The listing builds one solid part. Answer for the finished solid, in the listing's coordinates (mm). A direction names the side the tool comes from. Coordinates: 2 decimals unless noted, no trailing zeros. Order: outer loops, then holes, each group sorted by start corner. A loop starts at its lowest first (then second) coordinate and runs counter-clockwise, first axis right, second up. Notation, with made-up numbers: (9.5, 71) -> (45.5, 71) arc R12 ccw to (45.5, 93) -> close; hole circle Ø10 at (-28.75, 57). An arc over 180 degrees is marked (long way). Answer in a Markdown table with one row per item.
```python
from build123d import *

# Parameters (mm, degrees)
BOSS_EXTRUDE1_DEPTH = 19.5
SHELL1_T            = -3
SKETCH2_W           = 36
SKETCH2_H           = 39
CUT_EXTRUDE1_DEPTH  = 3
FILLET1_R           = 5
CUT_EXTRUDE2_REACH  = 41
SKETCH3_R           = 3


with BuildPart() as part:
    # Sketch1 → Boss-Extrude1 (new body, symmetric)
    with BuildSketch(Plane(origin=(0, 0, 0), x_dir=(1, 0, 0), z_dir=(0, 1, 0))):
        Polygon((0, -36), (0, -75), (-36, -75), (-39, -75), (-39, 75), (0, 75), (0, 0), align=None)
    boss_extrude1 = extrude(amount=BOSS_EXTRUDE1_DEPTH, both=True)

    # Mirror1: Boss-Extrude1 across plane
    add(boss_extrude1.mirror(Plane(origin=(0, 0, 0), x_dir=(0, 0, 1), z_dir=(1, 0, 0))))

    # Shell1
    shell1_openings = [part.faces().sort_by_distance(p)[0] for p in [
        (0, 0, 75),
        (0, 0, -75),
        (0, -19.5, 0),
    ]]
    offset(amount=SHELL1_T, openings=shell1_openings, kind=Kind.INTERSECTION)

    # Sketch2 → Cut-Extrude1 (cut)
    with BuildSketch(Plane(origin=(0, 19.5, 0), x_dir=(1, 0, 0), z_dir=(0, 1, 0))):
        with Locations((-18, -55.5)):
            Rectangle(SKETCH2_W, SKETCH2_H)
    cut_extrude1 = extrude(amount=-CUT_EXTRUDE1_DEPTH, mode=Mode.SUBTRACT)

    # Mirror2: Cut-Extrude1 across plane
    add(cut_extrude1.mirror(Plane(origin=(0, 0, 0), x_dir=(0, 0, 1), z_dir=(1, 0, 0))), mode=Mode.SUBTRACT)

    # Fillet1
    fillet1_edges = [part.edges().sort_by_distance(p)[0] for p in [
        (-37.5, 19.5, 75),
        (-37.5, -19.5, -75),
        (37.5, -19.5, 75),
        (37.5, 19.5, 75),
        (-37.5, -19.5, 75),
        (37.5, -19.5, -75),
    ]]
    fillet(fillet1_edges, radius=FILLET1_R)

    # Sketch3 → Cut-Extrude2 (cut, up to next)
    with BuildSketch(Plane(origin=(0, 19.5, 0), x_dir=(1, 0, 0), z_dir=(0, 1, 0)), mode=Mode.PRIVATE) as cut_extrude2_sk1:
        with Locations((-31, 67)):
            Circle(SKETCH3_R)
    cut_extrude2_tool1 = extrude(cut_extrude2_sk1.sketch, amount=-CUT_EXTRUDE2_REACH, mode=Mode.PRIVATE) & part.part
    add(cut_extrude2_tool1.solids().sort_by_distance((-31, 19.5, -67))[0], mode=Mode.SUBTRACT)
    # Sketch3 → Cut-Extrude2 (cut, up to next)
    with BuildSketch(Plane(origin=(0, 19.5, 0), x_dir=(1, 0, 0), z_dir=(0, 1, 0)), mode=Mode.PRIVATE) as cut_extrude2_sk2:
        with Locations((-31, -28)):
            Circle(SKETCH3_R)
    cut_extrude2_tool2 = extrude(cut_extrude2_sk2.sketch, amount=-CUT_EXTRUDE2_REACH, mode=Mode.PRIVATE) & part.part
    add(cut_extrude2_tool2.solids().sort_by_distance((-31, 19.5, 28))[0], mode=Mode.SUBTRACT)
    # Sketch3 → Cut-Extrude2 (cut, up to next)
    with BuildSketch(Plane(origin=(0, 19.5, 0), x_dir=(1, 0, 0), z_dir=(0, 1, 0)), mode=Mode.PRIVATE) as cut_extrude2_sk3:
        with Locations((11, -28)):
            Circle(SKETCH3_R)
    cut_extrude2_tool3 = extrude(cut_extrude2_sk3.sketch, amount=-CUT_EXTRUDE2_REACH, mode=Mode.PRIVATE) & part.part
    add(cut_extrude2_tool3.solids().sort_by_distance((11, 19.5, 28))[0], mode=Mode.SUBTRACT)
    # Sketch3 → Cut-Extrude2 (cut, up to next)
    with BuildSketch(Plane(origin=(0, 19.5, 0), x_dir=(1, 0, 0), z_dir=(0, 1, 0)), mode=Mode.PRIVATE) as cut_extrude2_sk4:
        with Locations((11, 67)):
            Circle(SKETCH3_R)
    cut_extrude2_tool4 = extrude(cut_extrude2_sk4.sketch, amount=-CUT_EXTRUDE2_REACH, mode=Mode.PRIVATE) & part.part
    add(cut_extrude2_tool4.solids().sort_by_distance((11, 19.5, -67))[0], mode=Mode.SUBTRACT)


solid = part.part
```
(1) A cutting plane is placed at B-B, the plane z = -67. Determine the outline of the cut face in (x, y), then the cut area to 3 significant figures.
Check values:
| item | result |
|---|---|
| outline | (-39, -19.5) -> (-36, -19.5) -> (-36, 16.5) -> (-34, 16.5) -> (-34, 19.5) -> (-39, 19.5) -> close; (-28, 16.5) -> (8, 16.5) -> (8, 19.5) -> (-28, 19.5) -> close; (14, 16.5) -> (36, 16.5) -> (36, -19.5) -> (39, -19.5) -> (39, 19.5) -> (14, 19.5) -> close |
| area | 414 mm² |
(2) For a pull along Z with two mould halves and no side action, classify faces 1 (the flat face through (38, 0, 75)), 2 (the cylindrical face through (-34, 18, 28)), 3 (the flat face through (-39, 0, 1)), 4 (the flat face through (3, 18, -75)) as released by +Z, released by -Z, zero draft, split by the parting line, or undercut.
Check values:
| item | result |
|---|---|
| face 1 | released by +Z |
| face 2 | undercut |
| face 3 | zero draft |
| face 4 | released by -Z |
(3) A cutting plane is placed at C-C, the plane y = -10. Determine the outline of the cut face in (x, z), then the cut area to 3 significant figures.
Check values:
| item | result |
|---|---|
| outline | (-39, -75) -> (-36, -75) -> (-36, 75) -> (-39, 75) -> close; (36, -75) -> (39, -75) -> (39, 75) -> (36, 75) -> close |
| area | 900 mm² |
(4) A cutting plane is placed at D-D, the plane z = 51. Determine the outline of the cut face in (x, y), then the cut area to 3 significant figures.
Check values:
| item | result |
|---|---|
| outline | (-39, -19.5) -> (-36, -19.5) -> (-36, 19.5) -> (-39, 19.5) -> close; (36, -19.5) -> (39, -19.5) -> (39, 19.5) -> (36, 19.5) -> close |
| area | 234 mm² |
(5) Flat-ended cylindrical pins translate along their axes: pin 1 (3.5 mm diameter, centred on x = -31, z = 28, fed in from +Y); pin 2 (6 mm diameter, centred on x = -14, z = 16, fed in from -Y); pin 3 (2.5 mm diameter, centred on x = 4.5, y = 18, fed in from +Z). Find the tip coordinate at first contact, or state that the pin passes through.
Check values:
| item | result |
|---|---|
| pin 1 | through |
| pin 2 | y = 16.5 |
| pin 3 | z = 36 |
(6) Find the intervals of material crossed by line 1 along X through (y, z) = (18.7, -67); line 2 along X through (y, z) = (-0.5, -43); line 3 along Y through (x, z) = (-34.5, 26), in increasing order. Write a range as from..to.
Check values:
| item | result |
|---|---|
| line 1 | -39..-34, -28..8, 14..39 |
| line 2 | -39..-36, 36..39 |
| line 3 | 16.5..19.5 |
(7) Which of the six approach directions +Z, -Z, +X, -X, +Y, -Y give full straight-line access (tool end or side, diameter ignored) to faces 5 (the flat face through (37, -19.5, -1)), 6 (the flat face through (1, 18, 36))?
Check values:
| item | result |
|---|---|
| face 5 | +Z, -Z, +X, -X, -Y |
| face 6 | +Z, +Y, -Y |
(8) A cutting plane is placed at A-A, the plane x = -31. Determine the outline of the cut face in (y, z), then the cut area to 3 significant figures.
Check values:
| item | result |
|---|---|
| outline | (16.5, -75) -> (19.5, -75) -> (19.5, -70) -> (16.5, -70) -> close; (16.5, -64) -> (19.5, -64) -> (19.5, 25) -> (16.5, 25) -> close; (16.5, 31) -> (19.5, 31) -> (19.5, 36) -> (16.5, 36) -> close |
| area | 297 mm² |
